Verification items for the finished model (mm, model axes). Round coordinates to 2 decimals unless told otherwise and drop trailing zeros. Loops run counter-clockwise (first coordinate to the right, second up) from the corner with the lowest first, then second, coordinate; pieces in that order, holes last. Notation, with made-up numbers: M -34,-33 L 4,-33 A7 cw 4,-20 Z; hole C 32.25,-27.75 d2. An arc over 180 degrees is marked long. Answer as CSV lines item,"result".
```python
from build123d import *

# Parameters (mm, degrees)
SKETCH_1_R          = 1.025
EXTRUDE_1_DEPTH     = 1.23
SKETCH_2_W          = 5.3
SKETCH_2_H          = 5.3
CUT_EXTRUDE_1_DEPTH = 10
FILLET_1_R          = 1.5


with BuildPart() as part:
    # 草图1 → 凸台-拉伸1 (new body)
    with BuildSketch(Plane.XY):
        with BuildLine():
            Line((44.125, 15.2), (44.125, -44.1))
            Line((44.125, -44.1), (40.475, -44.1))
            ThreePointArc((40.475, -44.1), (38.625, -45.95), (40.475, -47.8))
            Line((40.475, -47.8), (44.125, -47.8))
            Line((44.125, -47.8), (44.125, -52.85))
            ThreePointArc((44.125, -52.85), (39.731601718, -63.456601718), (29.125, -67.85))
            Line((29.125, -67.85), (-24.025, -67.85))
            Line((-24.025, -67.85), (-24.025, -58.75))
            Line((-24.025, -58.75), (-13.525, -58.75))
            Line((-13.525, -58.75), (-13.525, -38.65))
            Line((-13.525, -38.65), (-44.125, -38.65))
            Line((-44.125, -38.65), (-44.125, 15.2))
            Line((-44.125, 15.2), (-40.475, 15.2))
            ThreePointArc((-40.475, 15.2), (-38.625, 17.05), (-40.475, 18.9))
            Line((-40.475, 18.9), (-44.125, 18.9))
            Line((-44.125, 18.9), (-44.125, 67.85))
            Line((-44.125, 67.85), (44.125, 67.85))
            Line((44.125, 67.85), (44.125, 18.9))
            Line((44.125, 18.9), (40.475, 18.9))
            ThreePointArc((40.475, 18.9), (38.625, 17.05), (40.475, 15.2))
            Line((40.475, 15.2), (44.125, 15.2))
        make_face()
        with Locations((-22.025, -63)):
            Circle(SKETCH_1_R, mode=Mode.SUBTRACT)
        with Locations((-19.125, -10.6)):
            Circle(SKETCH_1_R, mode=Mode.SUBTRACT)
        with Locations((-0.025, -39.95)):
            Circle(SKETCH_1_R, mode=Mode.SUBTRACT)
        with Locations((-38.225, -33.65)):
            Circle(SKETCH_1_R, mode=Mode.SUBTRACT)
        with Locations((25.075, -37.55)):
            Circle(SKETCH_1_R, mode=Mode.SUBTRACT)
        with Locations((19.125, -10.6)):
            Circle(SKETCH_1_R, mode=Mode.SUBTRACT)
    extrude(amount=EXTRUDE_1_DEPTH)

    # 草图2 → 切除-拉伸1 (cut)
    with BuildSketch(Plane.XY.offset(1.23)):
        with Locations((-41.475, 65.2)):
            Rectangle(SKETCH_2_W, SKETCH_2_H)
        with Locations((41.475, 65.2)):
            Rectangle(SKETCH_2_W, SKETCH_2_H)
    extrude(amount=-CUT_EXTRUDE_1_DEPTH, mode=Mode.SUBTRACT)

    # 圆角1
    fillet_1_edges = [part.edges().sort_by_distance(p)[0] for p in [
        (-38.825, 62.55, 0.615),
        (38.825, 62.55, 0.615),
    ]]
    fillet(fillet_1_edges, radius=FILLET_1_R)


solid = part.part
```
1) Section check A-A (z = 0.55). State how many separate pieces and enclosed holes the cut face has, plus the area to 3 significant figures.
Here are the results:
separate pieces,"1"
enclosed holes,"6"
area,"11,000 mm^2"
2) Section check B-B (y = -45.95). Record the cut outline in (x, z) (3 decimals), plus the area to 3 significant figures.
Here are the results:
outline,"M -13.525,0 L 38.625,0 L 38.625,1.23 L -13.525,1.23 Z"
area,"64.1 mm^2"
3) Material ranges on probe 1 along X at (y, z) = (-10.5, 0.25) (3 decimals); probe 2 along Y at (x, z) = (-14, 0.7); probe 3 along X at (y, z) = (-11, 0.7) (3 decimals), recorded low to high.
Here are the results:
probe 1,"x = -44.125 to -20.145, -18.105 to 18.105, 20.145 to 44.125"
probe 2,"y = -67.85 to -58.75, -38.65 to 67.85"
probe 3,"x = -44.125 to -20.069, -18.181 to 18.181, 20.069 to 44.125"
4) Section check C-C (x = -31). Record the cut outline in (y, z).
Here are the results:
outline,"M -38.65,0 L 67.85,0 L 67.85,1.23 L -38.65,1.23 Z"
5) Go/stop test with a flat-tipped pin: pin 1 (0.6 mm diameter, centred on x = 41.5, z = 1, fed in from +Y). Record where the tip stops, or that it passes through.
Here are the results:
pin 1,"stops at y = 62.55"
